CAD build for the part. Positions are in the model's coordinates, mm. Face numbers are marked on the shaded views. A direction names the side the tool comes from. Round coordinates to 2 decimals unless told otherwise and drop trailing zeros. Write each loop counter-clockwise with the first axis right and the second up, starting at its lowest first coordinate (ties: lowest second). Pieces come first, ordered by that corner, then holes. Notation, with made-up numbers: (-13, 27.25) -> (13, 27.25) arc R37 cw to (13, 63.25) -> close; hole circle Ø8 at (48.25, -5). An arc over 180 degrees is marked (long way). Put each result on its own line as item: value. Start each with the question number.
1. 3-axis set-ups, long thin cutter, end or side, ignore diameter. For the marked faces 1 and 2: which of +Z, -Z, +X, -X, +Y, -Y reach the whole face in a straight line?
2. Saw through at C-C on y = 305.5. List the corners of the cut face in (x, z), and give its area (3 significant figures).
3. Flat gauge pins, fed straight in: P1, Ø3, axis at x = 795, y = 1072, coming from the +Z side; P2, Ø25, axis at x = 1081.5, z = 53.5, coming from the -Y side. Where does each tip first touch, or does it go through?
4. Drill centre lines: line 1 (Y direction, x = 1584, z = 58.5); line 2 (Z direction, x = 645, y = 851). Where is each one in solid material? Low to high. Write a range as from..to.
5. Saw through at B-B on z = 44.5. List the corners of the cut face in (x, y).
6. Saw through at A-A on x = 815. List the corners of the cut face in (y, z).
Autodesk Inventor part; units mm, degrees
ref_plane "YZ Plane" through (0, 0, 0) normal (1, 0, 0) x (0, 1, 0)
ref_plane "XZ Plane" through (0, 0, 0) normal (0, 1, 0) x (-1, 0, 0)
ref_plane "XY Plane" through (0, 0, 0) normal (0, 0, 1) x (1, 0, 0)
sketch "Szkic1" plane through (0, 0, 0) normal (0, 0, 1) x (1, 0, 0)
  line L0 (0, 0) -> (1800, 0)
  line L1 (1800, 0) -> (1800, 1700)
  line L2 (1800, 1700) -> (0, 1700)
  line L3 (0, 1700) -> (0, 0)
  line L4 (0, 1681) -> (1800, 1681)
  dimension "d0" = 1800
  dimension "d1" = 1700
  dimension "d2" = 19
extrude "Wyciągnięcie proste1" add sketch "Szkic1" along normal blind 69 contours L3 L2 L1 L4
extrude "Wyciągnięcie proste2" add sketch "Szkic1" along normal blind 19 contours L3 L4 L1 L0
properties part number "blat" material "Drewno (klon)"
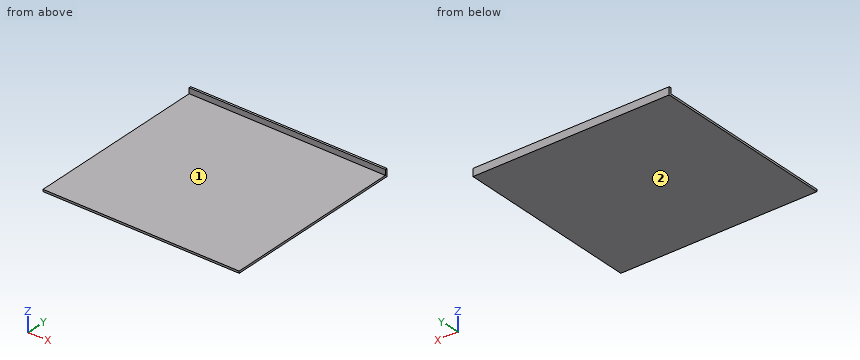
Return value:
1. face 1: +Z, +X, -X, -Y
1. face 2: -Z, +X, -X, +Y, -Y
2. outline: (0, 0) -> (1800, 0) -> (1800, 19) -> (0, 19) -> close
2. area: 34,200 mm^2
3. P1: stops at z = 19
3. P2: stops at y = 1681
4. line 1: y = 1681..1700
4. line 2: z = 0..19
5. outline: (0, 1681) -> (1800, 1681) -> (1800, 1700) -> (0, 1700) -> close
6. outline: (0, 0) -> (1700, 0) -> (1700, 69) -> (1681, 69) -> (1681, 19) -> (0, 19) -> close
